Autodesk Inventor part; units mm, degrees
ref_plane "YZ Plane" through (0, 0, 0) normal (1, 0, 0) x (0, 1, 0)
ref_plane "XZ Plane" through (0, 0, 0) normal (0, 1, 0) x (-1, 0, 0)
ref_plane "XY Plane" through (0, 0, 0) normal (0, 0, 1) x (1, 0, 0)
sketch "Skizze1" plane through (0, 0, 0) normal (0, 0, 1) x (1, 0, 0)
  circle A0 centre (0, 0) radius 2.3
  line L0 (-73.5, 5) -> (27, 5)
  line L1 (27, -39) -> (-73.5, -39)
  line L2 (-73.5, -39) -> (-73.5, 5)
  circle A1 centre (20, 0) radius 2.3
  circle A2 centre (0, -34) radius 2.3
  circle A3 centre (20, -34) radius 2.3
  line L3 (27, -29) -> (12, -29)
  line L4 (12, -29) -> (12, -5)
  line L5 (12, -5) -> (27, -5)
  line L6 (27, 5) -> (27, -5)
  line L7 (27, -29) -> (27, -39)
  dimension "d0" = 4.6
  dimension "d3" = 20
  dimension "d6" = 34
  dimension "d9" = 10
  dimension "d11" = 5
  dimension "d12" = 5
  dimension "d13" = 5
  dimension "d15" = 15
  dimension "d16" = 7
  dimension "d17" = 100.5
extrude "Extrusion1" add sketch "Skizze1" along normal blind 3
sketch "Skizze2" plane through (0, 0, 3) normal (0, 0, 1) x (1, 0, 0)
  circle A0 centre (-69.5, -34) radius 1.5
  circle A1 centre (20, -34) radius 2.3
  circle A2 centre (0, -34) radius 2.3
  circle A3 centre (20, 0) radius 2.3
  circle A4 centre (0, 0) radius 2.3
  line L0 (27, 5) -> (-73.5, 5)
  line L1 (-73.5, 5) -> (-73.5, -39)
  line L2 (-73.5, -39) -> (27, -39)
  line L3 (27, -39) -> (27, -29)
  line L4 (27, -29) -> (12, -29)
  line L5 (12, -29) -> (12, -5)
  line L6 (12, -5) -> (27, -5)
  line L7 (27, -5) -> (27, 5)
  circle A5 centre (-33.5, -34) radius 1.5
  circle A6 centre (-69.5, -22) radius 1.5
  circle A7 centre (-33.5, -22) radius 1.5
  dimension "d20" = 3
  dimension "d21" = 5
  dimension "d22" = 4
  dimension "d25" = 36
  dimension "d28" = 12
extrude "Extrusion2" cut sketch "Skizze2" against normal up to surface (3 mm away) contours A0 | A5 | A6 | A7
sketch "Skizze3" plane through (0, 0, 3) normal (0, 0, 1) x (1, 0, 0)
  circle A0 centre (-69.5, -22) radius 1.5
  circle A1 centre (-33.5, -22) radius 1.5
  circle A2 centre (-33.5, -34) radius 1.5
  circle A3 centre (-69.5, -34) radius 1.5
  circle A4 centre (20, -34) radius 2.3
  circle A5 centre (0, -34) radius 2.3
  circle A6 centre (20, 0) radius 2.3
  circle A7 centre (0, 0) radius 2.3
  line L0 (27, 5) -> (-73.5, 5)
  line L1 (-73.5, 5) -> (-73.5, -39)
  line L2 (-73.5, -39) -> (27, -39)
  line L3 (27, -39) -> (27, -29)
  line L4 (27, -29) -> (12, -29)
  line L5 (12, -29) -> (12, -5)
  line L6 (12, -5) -> (27, -5)
  line L7 (27, -5) -> (27, 5)
  line L8 (-73.5, 5) -> (-29.5, 5)
  line L9 (-29.5, 5) -> (-29.5, 5.1)
  line L10 (-29.5, 5.1) -> (-73.5, 5.1)
  line L11 (-73.5, 5.1) -> (-73.5, 5)
  line L12 (-53, 5.1) -> (-50, 5.1)
  line L13 (-50, 5.1) -> (-50, 115.1)
  line L14 (-50, 115.1) -> (-53, 115.1)
  line L15 (-53, 115.1) -> (-53, 5.1)
  line L16 (-58, 5.1) -> (-45, 5.1)
  line L17 (-45, 5.1) -> (-45, 120.1)
  line L18 (-45, 120.1) -> (-58, 120.1)
  line L19 (-58, 120.1) -> (-58, 5.1)
  line L20 (-73.5, 5.1) -> (-58, 50.1)
  line L21 (-29.5, 5.1) -> (-45, 50.1)
  dimension "d33" = 44
  dimension "d34" = 0.1
  dimension "d35" = 3
  dimension "d36" = 110
  dimension "d37" = 5
  dimension "d38" = 5
  dimension "d39" = 5
  dimension "d40" = 15.5
  dimension "d41" = 45
  dimension "d42" = 45
  dimension "d46" = 15.5
  dimension "d47" = 16.5
  dimension "d48" = 16.5
extrude "Extrusion3" add sketch "Skizze3" against normal up to surface (3 mm away) contours L0 L11 L10 L9 | L10 L17 L21 | L20 L19 L10 | L10 L13 L14 L15 L19 L18 L17
sketch "Skizze4" plane through (0, 0, 3) normal (0, 0, 1) x (1, 0, 0)
  line L0 (-53, 5.1) -> (-53, 115.1)
  line L1 (-53, 115.1) -> (-50, 115.1)
  line L2 (-50, 115.1) -> (-50, 5.1)
  line L3 (-50, 5.1) -> (-53, 5.1)
  circle A0 centre (-69.5, -22) radius 1.5
  circle A1 centre (-33.5, -22) radius 1.5
  circle A2 centre (-33.5, -34) radius 1.5
  circle A3 centre (-69.5, -34) radius 1.5
  circle A4 centre (20, -34) radius 2.3
  circle A5 centre (0, -34) radius 2.3
  circle A6 centre (20, 0) radius 2.3
  circle A7 centre (0, 0) radius 2.3
  line L4 (27, 5) -> (-29.5, 5)
  line L5 (-29.5, 5) -> (-29.5, 5.1)
  line L6 (-29.5, 5.1) -> (-45, 50.1)
  line L7 (-45, 50.1) -> (-45, 120.1)
  line L8 (-45, 120.1) -> (-58, 120.1)
  line L9 (-58, 120.1) -> (-58, 50.1)
  line L10 (-58, 50.1) -> (-73.5, 5.1)
  line L11 (-73.5, 5.1) -> (-73.5, -39)
  line L12 (-73.5, -39) -> (27, -39)
  line L13 (27, -39) -> (27, -29)
  line L14 (27, -29) -> (12, -29)
  line L15 (12, -29) -> (12, -5)
  line L16 (12, -5) -> (27, -5)
  line L17 (27, -5) -> (27, 5)
  arc A8 (-50, 115.1) -> (-53, 115.1) centre (-51.5, 115.1) ccw
  line L18 (-50, 5.1) -> (-53, 5.1)
  arc A9 (-53, 5.1) -> (-50, 5.1) centre (-51.5, 5.1) ccw
extrude "Extrusion4" cut sketch "Skizze4" against normal up to surface (3 mm away) contours L3 A9 | A8 L1
sketch "Skizze6" plane through (0, 0, 3) normal (0, 0, 1) x (1, 0, 0)
  line L0 (27, 5) -> (-29.5, 5)
  line L1 (-29.5, 5) -> (-29.5, 5.1)
  line L2 (-29.5, 5.1) -> (-45, 50.1)
  line L3 (-45, 50.1) -> (-45, 120.1)
  line L4 (-45, 120.1) -> (-58, 120.1)
  line L5 (-58, 120.1) -> (-58, 50.1)
  line L6 (-58, 50.1) -> (-73.5, 5.1)
  line L7 (-73.5, 5.1) -> (-73.5, -39)
  line L8 (-73.5, -39) -> (27, -39)
  line L9 (27, -39) -> (27, -29)
  line L10 (27, -29) -> (12, -29)
  line L11 (12, -29) -> (12, -5)
  line L12 (12, -5) -> (27, -5)
  line L13 (27, -5) -> (27, 5)
  circle A0 centre (0, 0) radius 2.3
  circle A1 centre (20, 0) radius 2.3
  circle A2 centre (0, -34) radius 2.3
  circle A3 centre (20, -34) radius 2.3
  circle A4 centre (-69.5, -34) radius 1.5
  circle A5 centre (-33.5, -34) radius 1.5
  circle A6 centre (-33.5, -22) radius 1.5
  circle A7 centre (-69.5, -22) radius 1.5
  arc A8 (-53, 5.1) -> (-50, 5.1) centre (-51.5, 5.1) ccw
  line L14 (-53, 5.1) -> (-53, 115.1)
  arc A9 (-50, 115.1) -> (-53, 115.1) centre (-51.5, 115.1) ccw
  line L15 (-50, 115.1) -> (-50, 5.1)
properties part number "Upper_plate"
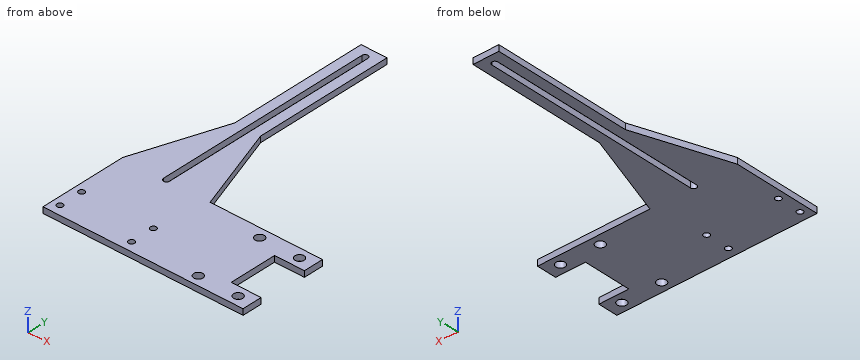
Design review of the part built by this model. Coordinates are the model's own, in mm. Give positions to 0.01 mm unless a question says otherwise; leave off trailing zeros. Loops run counter-clockwise (first coordinate to the right, second up) from the corner with the lowest first, then second, coordinate; pieces in that order, holes last. Notation, with made-up numbers: (50.5, -25) - (84.5, -25) arc R28 cw to (84.5, -2) - close; hole circle Ø8 at (80.5, 85.25). An arc over 180 degrees is marked (long way). Use CSV: the item, a comma, the result in double quotes. Start each with the question number.
1. Add section C-C (y = 103.5). State the section outline as (x, z) points, plus the area to 3 significant figures.
2. Add section D-D (z = 1). Count the separate pieces of the cut face and the enclosed holes in it, plus the area to 3 significant figures.
3. Add section B-B (x = 20). State the section outline as (y, z) points, plus the area to 3 significant figures.
4. Insertion check: P1, Ø2.5, axis at x = -33.5, y = -34, coming from the -Z side; P2, Ø0.9, axis at y = -11.5, z = 2, coming from the +X side; P3, Ø1.5, axis at y = 40, z = 2, coming from the +X side. Each pin has a flat end and moves straight along its axis. Give the tip position at first contact, or say it passes through.
5. Wall thickness on L1, parallel to Y at x = 20, z = 2.3; L2, parallel to X at y = 99, z = 1.2; L3, parallel to Y at x = 0, z = 0.65: over which ranges is each line inside the solid? List them lowest first.
6. Add section A-A (y = 0). State the section outline as (x, z) points.
Results found:
1,outline,"(-58, 0) - (-53, 0) - (-53, 3) - (-58, 3) - close; (-50, 0) - (-45, 0) - (-45, 3) - (-50, 3) - close"
1,area,"30.0 mm²"
2,separate pieces,"1"
2,enclosed holes,"9"
2,area,"5,830 mm²"
3,outline,"(-39, 0) - (-36.3, 0) - (-36.3, 3) - (-39, 3) - close; (-31.7, 0) - (-29, 0) - (-29, 3) - (-31.7, 3) - close; (-5, 0) - (-2.3, 0) - (-2.3, 3) - (-5, 3) - close; (2.3, 0) - (5, 0) - (5, 3) - (2.3, 3) - close"
3,area,"32.4 mm²"
4,P1,"passes through"
4,P2,"stops at x = 12"
4,P3,"stops at x = -41.26"
5,L1,"y = -39 to -36.3, -31.7 to -29, -5 to -2.3, 2.3 to 5"
5,L2,"x = -58 to -53, -50 to -45"
5,L3,"y = -39 to -36.3, -31.7 to -2.3, 2.3 to 5"
6,outline,"(-73.5, 0) - (-2.3, 0) - (-2.3, 3) - (-73.5, 3) - close; (2.3, 0) - (17.7, 0) - (17.7, 3) - (2.3, 3) - close; (22.3, 0) - (27, 0) - (27, 3) - (22.3, 3) - close"
